from build123d import *

# Parameters (mm, degrees)
ESQUISSE1_W                     = 81
ESQUISSE1_H                     = 61
ESQUISSE1_W_2                   = 65
ESQUISSE1_H_2                   = 45
EXTRU_MINCE1_DEPTH              = 4
ESQUISSE3_R                     = 1
ENL_V_MAT_EXTRU_1_DEPTH         = 13
ESQUISSE4_W                     = 81
ESQUISSE4_H                     = 61
ESQUISSE4_W_2                   = 76
ESQUISSE4_H_2                   = 56
EXTRU_MINCE2_DEPTH              = 12
ENL_V_MAT_EXTRU_5_DEPTH         = 11.5
ENL_V_MAT_EXTRU_4_DEPTH         = 1.5
ESQUISSE9_W                     = 78
ESQUISSE9_H                     = 58
ESQUISSE9_W_2                   = 76
ESQUISSE9_H_2                   = 56
ENL_V_DE_MAT_EXTRU_MINCE1_DEPTH = 2.5
CONG_4_R                        = 1
CONG_5_R                        = 2


with BuildPart() as part:
    # Esquisse1 → Extru.-Mince1 (new body)
    with BuildSketch(Plane.XY):
        with Locations((32.5, 22.5)):
            Rectangle(ESQUISSE1_W, ESQUISSE1_H)
        with Locations((32.5, 22.5)):
            Rectangle(ESQUISSE1_W_2, ESQUISSE1_H_2, mode=Mode.SUBTRACT)
    extrude(amount=EXTRU_MINCE1_DEPTH)

    # Esquisse3 → Enlèv. mat.-Extru.1 (cut)
    with BuildSketch(Plane.XY):
        with Locations((-2.5, 33)):
            Circle(ESQUISSE3_R)
        with Locations((-2.5, 12)):
            Circle(ESQUISSE3_R)
        with Locations((67.5, 33)):
            Circle(ESQUISSE3_R)
        with Locations((67.5, 12)):
            Circle(ESQUISSE3_R)
        Polygon((-0.11, 47.36), (19.39, 47.36), (19.39, 43.36), (19.39, 1.64), (19.39, -2.36), (-0.11, -2.36), (-0.11, 1.64), (-0.11, 43.36), align=None)
    extrude(amount=ENL_V_MAT_EXTRU_1_DEPTH, mode=Mode.SUBTRACT)

    # Esquisse4 → Extru.-Mince2 (add)
    with BuildSketch(Plane.XY):
        with Locations((32.5, 22.5)):
            Rectangle(ESQUISSE4_W, ESQUISSE4_H)
        with Locations((32.5, 22.5)):
            Rectangle(ESQUISSE4_W_2, ESQUISSE4_H_2, mode=Mode.SUBTRACT)
    extrude(amount=EXTRU_MINCE2_DEPTH)

    # Esquisse7 → Enlèv. mat.-Extru.5 (cut)
    with BuildSketch(Plane(origin=(-5.5, 0, 0), x_dir=(0, 0, -1), z_dir=(1, 0, 0))):
        with BuildLine():
            Line((-12, 42.802969616), (-12, 36.302969616))
            ThreePointArc((-12, 36.302969616), (-8.75, 39.552969616), (-12, 42.802969616))
        make_face()
    extrude(amount=-ENL_V_MAT_EXTRU_5_DEPTH, mode=Mode.SUBTRACT)

    # Esquisse6 → Enlèv. mat.-Extru.4 (cut)
    with BuildSketch(Plane(origin=(-5.5, 0, 0), x_dir=(0, 0, -1), z_dir=(1, 0, 0))):
        with BuildLine():
            Line((-12, 44.052969616), (-12, 35.052969616))
            ThreePointArc((-12, 35.052969616), (-7.5, 39.552969616), (-12, 44.052969616))
        make_face()
    extrude(amount=-ENL_V_MAT_EXTRU_4_DEPTH, mode=Mode.SUBTRACT)

    # Esquisse9 → Enlèv. de mat.-Extru.-Mince1 (cut)
    with BuildSketch(Plane.XY.offset(12)):
        with Locations((32.5, 22.5)):
            Rectangle(ESQUISSE9_W, ESQUISSE9_H)
        with Locations((32.5, 22.5)):
            Rectangle(ESQUISSE9_W_2, ESQUISSE9_H_2, mode=Mode.SUBTRACT)
    extrude(amount=-ENL_V_DE_MAT_EXTRU_MINCE1_DEPTH, mode=Mode.SUBTRACT)

    # Congé4
    cong_4_edges = [part.edges().sort_by_distance(p)[0] for p in [
        (-5.5, 50.5, 6.75),
        (70.5, 50.5, 6.75),
        (70.5, -5.5, 6.75),
        (-5.5, -5.5, 6.75),
    ]]
    fillet(cong_4_edges, radius=CONG_4_R)

    # Congé5
    cong_5_edges = [part.edges().sort_by_distance(p)[0] for p in [
        (-8, 53, 6),
        (73, 53, 6),
        (73, -8, 6),
        (-8, -8, 6),
    ]]
    fillet(cong_5_edges, radius=CONG_5_R)


solid = part.part
The listing builds one solid part. Answer for the finished solid, in the listing's coordinates (mm). A direction names the side the tool comes from. Round coordinates to 2 decimals unless told otherwise and drop trailing zeros. Write each loop counter-clockwise with the first axis right and the second up, starting at its lowest first coordinate (ties: lowest second). Pieces come first, ordered by that corner, then holes. Notation, with made-up numbers: M -32,1 L -19,1 A20 cw -19,18 Z; hole C -15,-31 d2. An arc over 180 degrees is marked long. Write each question's results on one line, items separated by ' | '. Start each with the question number.
Item 1: For a pull along X with two mould halves and no side action, classify faces 1 (the face through (72.43, 52.4, 5.92)), 2 (the face through (66.763, 33.676, 1.972)), 3 (the face through (-6.4, 39.5, 7.5)), 4 (the face through (-7, 23, 12)) as pulls with the +X half, pulls with the -X half, needs draft (parallel to the pull), parting line crosses it, or undercut.
Item 2: Flat-ended cylindrical pins translate along their axes: pin 1 Ø10 at (x, y) = (15.5, 5.5) entering from +Z (3 decimals); pin 2 Ø2.5 at (x, y) = (-2.5, 12) entering from +Z. Find the tip coordinate at first contact, or state that the pin passes through.
Item 3: A cutting plane is placed at B-B on y = 12. Write down the section's boundary in (x, z).
Item 4: A cutting plane is placed at D-D on y = 5. Write down the section's boundary in (x, z), and give its area (3 significant figures).
Item 5: Straight lines are drawn through the part: L1, parallel to Y at x = 67.5, z = 2.7; L2, parallel to X at y = 33, z = 2.6; L3, parallel to X at y = 3, z = 8. For each, find the intervals that lie inside material, in ascending order. Write a range as [from, to].
Item 6: A cutting plane is placed at A-A on x = 64. Write down the section's boundary in (y, z), and give its area (3 significant figures).
Item 7: For faces 5 (the face through (73, 22, 6)), 6 (the face through (32, 51.5, 11)), 7 (the face through (-7.49, 39.48, 8.75)), 8 (the face through (10, -2.36, 2)), determine the directions among +Z, -Z, +X, -X, +Y, -Y from which every point of the face is accessible in a straight line to the end or side of a thin tool.
Item 8: A cutting plane is placed at C-C on z = 3. Write down the section's boundary in (x, y), and give its area (3 significant figures).
Check sheet entries:
1) face 1: pulls with the +X half | face 2: undercut | face 3: undercut | face 4: needs draft
2) pin 1: through | pin 2: z = 4
3) outline: M -8,0 L -3.5,0 L -3.5,4 L -5.5,4 L -5.5,9.5 L -6.5,9.5 L -6.5,12 L -8,12 Z; M -1.5,0 L -0.11,0 L -0.11,4 L -1.5,4 Z; M 65,0 L 66.5,0 L 66.5,4 L 65,4 Z; M 68.5,0 L 73,0 L 73,12 L 71.5,12 L 71.5,9.5 L 70.5,9.5 L 70.5,4 L 68.5,4 Z
4) outline: M -8,0 L -0.11,0 L -0.11,4 L -5.5,4 L -5.5,9.5 L -6.5,9.5 L -6.5,12 L -8,12 Z; M 65,0 L 73,0 L 73,12 L 71.5,12 L 71.5,9.5 L 70.5,9.5 L 70.5,4 L 65,4 Z | area: 98.6 mm²
5) L1: [-8, 11], [13, 32], [34, 53] | L2: [-8, -3.5], [-1.5, -0.11], [65, 66.5], [68.5, 73] | L3: [-8, -5.5], [70.5, 73]
6) outline: M -8,0 L 0,0 L 0,4 L -5.5,4 L -5.5,9.5 L -6.5,9.5 L -6.5,12 L -8,12 Z; M 45,0 L 53,0 L 53,12 L 51.5,12 L 51.5,9.5 L 50.5,9.5 L 50.5,4 L 45,4 Z | area: 99.0 mm²
7) face 5: +Z, -Z, +X, +Y, -Y | face 6: +Z | face 7: +Z, -X | face 8: +Z, -Z
8) outline: M -8,-6 A2 ccw -6,-8 L 71,-8 A2 ccw 73,-6 L 73,51 A2 ccw 71,53 L -6,53 A2 ccw -8,51 Z; hole C -2.5,12 d2; hole C -2.5,33 d2; hole M -0.11,-2.36 L 19.39,-2.36 L 19.39,0 L 65,0 L 65,45 L 19.39,45 L 19.39,47.36 L -0.11,47.36 Z; hole C 67.5,12 d2; hole C 67.5,33 d2 | area: 1,900 mm²
